Part model, mm, in its own coordinate system. A direction names the side the tool comes from. Coordinates: 2 decimals unless noted, no trailing zeros. Order: outer loops, then holes, each group sorted by start corner. A loop starts at its lowest first (then second) coordinate and runs counter-clockwise, first axis right, second up.
from build123d import *

# Parameters (mm, degrees)
EXTRUDE_1_DEPTH     = 6
CUT_EXTRUDE_1_DEPTH = 3


with BuildPart() as part:
    # Эскиз1 → Бобышка-Вытянуть1 (new body)
    with BuildSketch(Plane(origin=(0, 0, 0), x_dir=(1, 0, 0), z_dir=(0, 1, 0))):
        with BuildLine():
            Line((-6, -3.75), (-6, 0))
            ThreePointArc((-6, 0), (0, 6), (6, 0))
            Line((6, 0), (6, -3.75))
            ThreePointArc((6, -3.75), (30.366066361, -18.254309704), (31.5, 10.079316686))
            Line((31.5, 10.079316686), (31.5, 22.23557292))
            ThreePointArc((31.5, 22.23557292), (44.461534369, -20.301163348), (0, -19.561388301))
            ThreePointArc((0, -19.561388301), (-44.461534369, -20.301163348), (-31.5, 22.23557292))
            Line((-31.5, 22.23557292), (-31.5, 10.079316686))
            ThreePointArc((-31.5, 10.079316686), (-30.366066361, -18.254309704), (-6, -3.75))
        make_face()
    extrude(amount=EXTRUDE_1_DEPTH)

    # Эскиз4 → Вырез-Вытянуть1 (cut)
    with BuildSketch(Plane(origin=(0, 6, 0), x_dir=(1, 0, 0), z_dir=(0, 1, 0))):
        with BuildLine():
            Line((-3.5, -3.75), (-3.5, 0))
            ThreePointArc((-3.5, 0), (0, 3.5), (3.5, 0))
            Line((3.5, 0), (3.5, -3.75))
            ThreePointArc((3.5, -3.75), (29.75403121, -20.546577032), (34, 10.33012784))
            Line((34, 10.33012784), (34, 17.034609691))
            ThreePointArc((34, 17.034609691), (37.989980812, -21.647500207), (0, -13.341663047))
            ThreePointArc((0, -13.341663047), (-37.989980812, -21.647500207), (-34, 17.034609691))
            Line((-34, 17.034609691), (-34, 10.33012784))
            ThreePointArc((-34, 10.33012784), (-29.75403121, -20.546577032), (-3.5, -3.75))
        make_face()
    extrude(amount=-CUT_EXTRUDE_1_DEPTH, mode=Mode.SUBTRACT)


solid = part.part
Q1. Cut at B-B on z = 25.5. Write the cut outline in (x, y), and give its area (3 significant figures).
Results list:
outline: (-39.33, 0) - (-5.67, 0) - (-5.67, 6) - (-11.85, 6) - (-11.85, 3) - (-32.15, 3) - (-32.15, 6) - (-39.33, 6) - close; (5.67, 0) - (39.33, 0) - (39.33, 6) - (32.15, 6) - (32.15, 3) - (11.85, 3) - (11.85, 6) - (5.67, 6) - close
area: 282 mm2
Q2. Cut at A-A on z = 5.5. Write the cut outline in (x, y), and give its area (3 significant figures).
Results list:
outline: (-49.94, 0) - (-38.91, 0) - (-38.91, 6) - (-40.42, 6) - (-40.42, 3) - (-45.94, 3) - (-45.94, 6) - (-49.94, 6) - close; (-6.09, 0) - (6.09, 0) - (6.09, 6) - (3.58, 6) - (3.58, 3) - (-3.58, 3) - (-3.58, 6) - (-6.09, 6) - close; (38.91, 0) - (49.94, 0) - (49.94, 6) - (45.94, 6) - (45.94, 3) - (40.42, 3) - (40.42, 6) - (38.91, 6) - close
area: 151 mm2
Q3. Wall check: line 1 along X through (y, z) = (2.3, 17); line 2 along X through (y, z) = (1.6, 12.5); line 3 along X through (y, z) = (5.3, 10). Give the ranges that are in metal, low to high.
Results list:
line 1: x = -46.6 to -32.33, -12.67 to 12.67, 32.33 to 46.6
line 2: x = -48.57 to -36.49, -8.51 to 8.51, 36.49 to 48.57
line 3: x = -49.28 to -45.17, -39.41 to -37.77, -7.23 to -4.59, 4.59 to 7.23, 37.77 to 39.41, 45.17 to 49.28
Q4. Which spindle directions (+Z, -Z, +X, -X, +Y, -Y) get a long thin tool onto all of the face, cutting with end or side? Do faces 1 (the face through (4, 6, 4)), 2 (the face through (34, 5, -14)), 3 (the face through (-31.5, 3, -16)). Say none if no direction does.
Results list:
face 1: +Z, -Z, +X, -X, +Y
face 2: +Y
face 3: -Z, +Y, -Y
Q5. Cut at D-D on x = 22. Write the cut outline in (y, z), and give its area (3 significant figures).
Results list:
outline: (0, 20.24) - (6, 20.24) - (6, 22.25) - (3, 22.25) - (3, 27.75) - (6, 27.75) - (6, 31.25) - (0, 31.25) - close
area: 49.5 mm2
Q6. Cut at C-C on y = 4.95. Write the cut outline in (x, z).
Results list:
outline: (-31.5, -22.24) - (-31.5, -10.08) arc R16.5 cw (long way) to (-6, 3.75) - (-6, 0) arc R6 ccw to (6, 0) - (6, 3.75) arc R16.5 cw (long way) to (31.5, -10.08) - (31.5, -22.24) arc R27.5 ccw (long way) to (0, 19.56) arc R27.5 ccw (long way) to start; hole (-34, -17.03) - (-34, -10.33) arc R18.5 cw (long way) to (-3.5, 3.75) - (-3.5, 0) arc R3.5 ccw to (3.5, 0) - (3.5, 3.75) arc R18.5 cw (long way) to (34, -10.33) - (34, -17.03) arc R24 ccw (long way) to (0, 13.34) arc R24 ccw (long way) to start
Q7. Pin check, flat tips, straight feed: pin 1 Ø0.9 at (y, z) = (4, -13.5) entering from -X; pin 2 Ø12 at (x, z) = (0.5, 6) entering from +Y; pin 3 Ø2 at (x, y) = (36.5, 5) entering from -Z; pin 4 Ø2.5 at (y, z) = (4.5, 1) entering from -X. Stop position of each tip, or through.
Results list:
pin 1: stops at x = -44.27
pin 2: stops at y = 6
pin 3: stops at z = -20.48
pin 4: stops at x = -49.96
Q8. Mould opens along Z. For faces 4 (the face through (29.943, 2.958, 18.476)), 5 (the face through (6, 3, 2)), 6 (the face through (44.9, 3, 19.7)) say: pulls with the +Z half, pulls with the -Z half, needs draft (parallel to the pull), parting line crosses it, or undercut.
Results list:
face 4: undercut
face 5: needs draft
face 6: parting line crosses it
